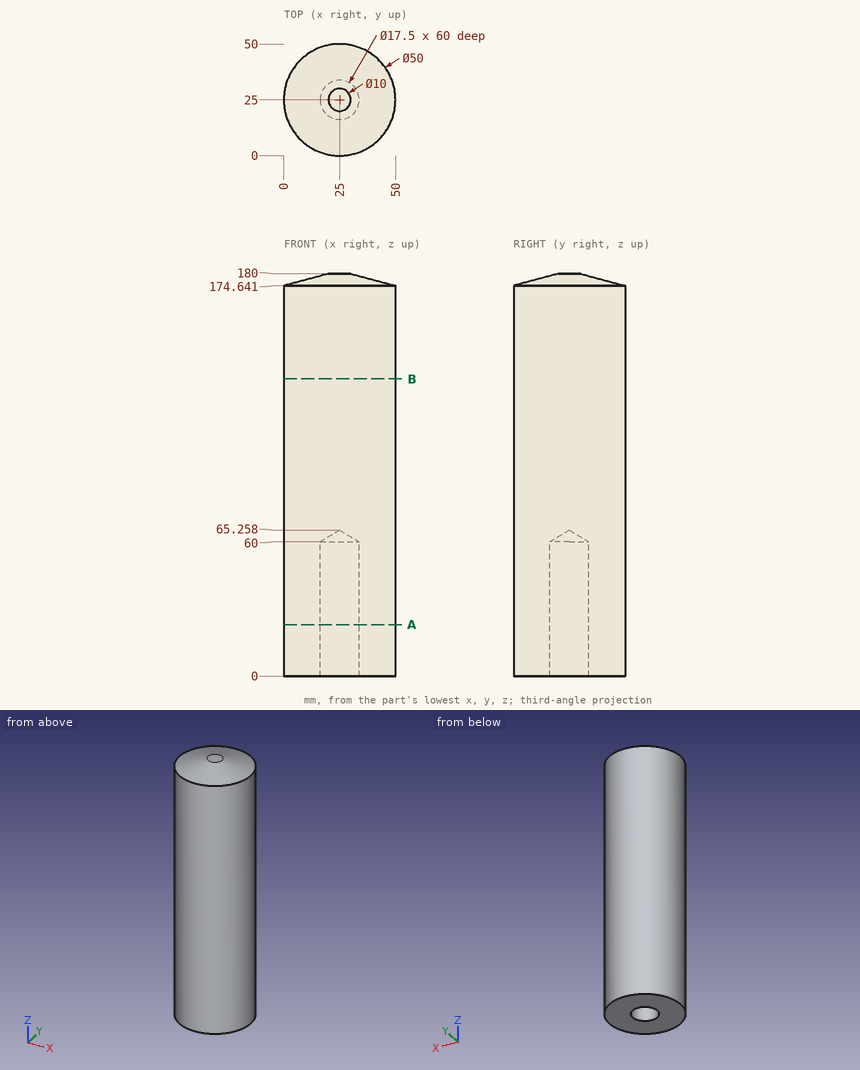
Here's the drawing with two shaded views (mm, measured from the low corner). I have some questions. Coordinates: 2 decimals unless noted, no trailing zeros. Order: outer loops, then holes, each group sorted by start corner. A loop starts at its lowest first (then second) coordinate and runs counter-clockwise, first axis right, second up.
Q1. Please list where these lines run through material, in increasing order: L1, parallel to Y at x = 25, z = 25; L2, parallel to X at y = 18, z = 10.5; L3, parallel to X at y = 22, z = 15.5.
Q2. Suppose I cut it at A-A on z = 23. Please give me the cut outline in (x, y).
Q3. Will these pins go through, and if not, where does the flat tip stop? pin 1 (14 mm diameter, centred on x = 25, y = 25, fed in from -Z); pin 2 (1.5 mm diameter, centred on y = 30.5, z = 45, fed in from +X) (1 decimal); pin 3 (3 mm diameter, centred on x = 40.5, y = 18, fed in from +Z) (1 decimal).
Q4. Suppose I cut it at B-B on z = 133. Please give me the cut outline in (x, y), and give its area (3 significant figures).
Answer:
1. L1: y = 0 to 16.25, 33.75 to 50
1. L2: x = 1 to 19.75, 30.25 to 49
1. L3: x = 0.18 to 16.78, 33.22 to 49.82
2. outline: circle Ø50 at (25, 25); hole circle Ø17.5 at (25, 25)
3. pin 1: stops at z = 61.05
3. pin 2: stops at x = 49.5
3. pin 3: stops at z = 177.2
4. outline: circle Ø50 at (25, 25)
4. area: 1,960 mm2
